```python
from build123d import *

# Parameters (mm, degrees)
CUT_EXTRUDE_1_DEPTH      = 5
EXTRUDE_1_DEPTH          = 6
PATTERN_CIRCULAR_1_COUNT = 3
SKETCH_4_R               = 42.404307435
SKETCH_4_R_2             = 25.5
CUT_EXTRUDE_2_DEPTH      = 9.5
CHAMFER_START            = 14
CHAMFER_1_DEPTH          = 6


with BuildPart() as part:
    # Эскиз1 → Повернуть1 (revolve)
    with BuildSketch(Plane.XY, mode=Mode.PRIVATE) as revolve_1_sk:
        with BuildLine():
            Line((-24, 0), (-24, 4.5))
            Line((-24, 4.5), (-25.5, 4.5))
            Line((-25.5, 4.5), (-25.5, 9.5))
            Line((-25.5, 9.5), (-19, 9.5))
            Line((-19, 9.5), (-19, 22))
            Line((-19, 22), (-24, 22))
            Line((-24, 22), (-24, 12.5))
            Line((-24, 12.5), (-27.5, 12.5))
            ThreePointArc((-27.5, 12.5), (-28.207106781, 12.207106781), (-28.5, 11.5))
            Line((-28.5, 11.5), (-28.5, 0))
            Line((-28.5, 0), (-24, 0))
        make_face()
    revolve(revolve_1_sk.sketch.rotate(Axis((0, 0, 0), (0, -1, 0)), 270), axis=Axis((0, 0, 0), (0, -1, 0)))

    # Эскиз2 → Вырез-Вытянуть1 (cut)
    with BuildSketch(Plane(origin=(0, 0, 0), x_dir=(-1, 0, 0), z_dir=(0, -1, 0))):
        with BuildLine():
            ThreePointArc((24, 0), (17.8818714, -16.007456864), (2.646777063, -23.85360709))
            Line((2.646777063, -23.85360709), (5, -25.514701644))
            ThreePointArc((5, -25.514701644), (20.0748599, -16.522711642), (26, 0))
            ThreePointArc((26, 0), (25.646694472, 4.271658071), (24.596379794, 8.427223803))
            Line((24.596379794, 8.427223803), (21.981218243, 9.63462737))
            ThreePointArc((21.981218243, 9.63462737), (23.489883331, 4.921928594), (24, 0))
        make_face()
        with BuildLine():
            Line((-5, -25.514701644), (-2.646777063, -23.85360709))
            ThreePointArc((-2.646777063, -23.85360709), (-20.784609691, -12), (-21.981218243, 9.63462737))
            Line((-21.981218243, 9.63462737), (-24.596379794, 8.427223803))
            ThreePointArc((-24.596379794, 8.427223803), (-22.516660498, -13), (-5, -25.514701644))
        make_face()
        with BuildLine():
            Line((-19.596379794, 17.087477841), (-19.33444118, 14.218979719))
            ThreePointArc((-19.33444118, 14.218979719), (0, 24), (19.33444118, 14.218979719))
            Line((19.33444118, 14.218979719), (19.596379794, 17.087477841))
            ThreePointArc((19.596379794, 17.087477841), (0, 26), (-19.596379794, 17.087477841))
        make_face()
    extrude(amount=-CUT_EXTRUDE_1_DEPTH, mode=Mode.SUBTRACT)

    # Эскиз3 → Бобышка-Вытянуть1 (add)
    with BuildSketch(Plane(origin=(25.5, 0, 0), x_dir=(0, 0, -1), z_dir=(1, 0, 0))):
        Polygon((-11.5, 20), (11.5, 20), (11.5, 17), (-11.5, 15), align=None)
    extrude_1 = extrude(amount=-EXTRUDE_1_DEPTH)

    # Круговой массив1: Бобышка-Вытянуть1 ×3 about axis
    pattern_circular_1_axis = Axis((0, 0, 0), (0, 1, 0))
    for i in range(1, PATTERN_CIRCULAR_1_COUNT):
        add(extrude_1.rotate(pattern_circular_1_axis, i * 360 / PATTERN_CIRCULAR_1_COUNT))

    # Эскиз4 → Вырез-Вытянуть2 (cut)
    with BuildSketch(Plane(origin=(0, 22, 0), x_dir=(1, 0, 0), z_dir=(0, 1, 0))):
        Circle(SKETCH_4_R)
        with Locations(Location((0, 0, 0), (0, 0, 270))):
            Circle(SKETCH_4_R_2, mode=Mode.SUBTRACT)
    extrude(amount=-CUT_EXTRUDE_2_DEPTH, mode=Mode.SUBTRACT)

    # Фаска1: read off the stored shape, not the designer's step
    # Фаска1 outline → Фаска1 (cut)
    with BuildSketch(Plane(origin=(0, 0, 0), x_dir=(1, 0, 0), z_dir=(0, 1, 0)).offset(CHAMFER_START)):
        with BuildLine():
            Line((-20.456443185, 12.551252218), (-20.356857991, 15.357354354))
            ThreePointArc((-20.356857991, 15.357354354), (-20.859675731, 14.667103612), (-21.33909882, 13.960403344))
            Line((-21.33909882, 13.960403344), (-20.49197936, 12.493149399))
            ThreePointArc((-20.49197936, 12.493149399), (-20.474231883, 12.522213414), (-20.456443185, 12.551252218))
        make_face()
        with BuildLine():
            ThreePointArc((-1.420514533, 25.460403344), (-2.272246462, 25.398560904), (-3.12143001, 25.308233338))
            Line((-3.12143001, 25.308233338), (-0.641481678, 23.991425578))
            ThreePointArc((-0.641481678, 23.991425578), (-0.607438987, 23.992311641), (-0.573395073, 23.993149399))
            Line((-0.573395073, 23.993149399), (-1.420514533, 25.460403344))
        make_face()
        with BuildLine():
            ThreePointArc((-20.456443185, -12.551252218), (-20.474231883, -12.522213414), (-20.49197936, -12.493149399))
            Line((-20.49197936, -12.493149399), (-21.33909882, -13.960403344))
            ThreePointArc((-21.33909882, -13.960403344), (-20.859675731, -14.667103612), (-20.356857991, -15.357354354))
            Line((-20.356857991, -15.357354354), (-20.456443185, -12.551252218))
        make_face()
        with BuildLine():
            Line((22.759613353, 11.5), (21.065374433, 11.5))
            ThreePointArc((21.065374433, 11.5), (21.08167087, 11.470098227), (21.097924862, 11.44017336))
            Line((21.097924862, 11.44017336), (23.478288, 9.950878984))
            ThreePointArc((23.478288, 9.950878984), (23.131922194, 10.731457292), (22.759613353, 11.5))
        make_face()
        with BuildLine():
            ThreePointArc((-0.573395073, -23.993149399), (-0.607438987, -23.992311641), (-0.641481678, -23.991425578))
            Line((-0.641481678, -23.991425578), (-3.12143001, -25.308233338))
            ThreePointArc((-3.12143001, -25.308233338), (-2.272246462, -25.398560904), (-1.420514533, -25.460403344))
            Line((-1.420514533, -25.460403344), (-0.573395073, -23.993149399))
        make_face()
        with BuildLine():
            ThreePointArc((22.759613353, -11.5), (23.131922194, -10.731457292), (23.478288, -9.950878984))
            Line((23.478288, -9.950878984), (21.097924862, -11.44017336))
            ThreePointArc((21.097924862, -11.44017336), (21.08167087, -11.470098227), (21.065374433, -11.5))
            Line((21.065374433, -11.5), (22.759613353, -11.5))
        make_face()
    extrude(amount=CHAMFER_1_DEPTH, mode=Mode.SUBTRACT)


solid = part.part
```
Read the model definition and answer for the solid it produces. Units are mm, in the model's axes. A direction names the side the tool comes from. Round coordinates to 2 decimals unless told otherwise and drop trailing zeros. One line per item, written item: value.
Q1. Which of the six approach directions +Z, -Z, +X, -X, +Y, -Y give full straight-line access (tool end or side, diameter ignored) to faces 5 (the flat face through (-12.3, 16, 21.3)), 6 (the cylindrical face through (-12.626, 18.142, -22.155)), 7 (the cylindrical face through (0, 2, 24)), 8 (the flat face through (0, 4.5, 25))?
Data:
face 5: +Z
face 6: -Z, -X, +Y
face 7: -Y
face 8: none
Q2. Straight lines are drawn through the part: line 1 (X direction, y = 15.5, z = 0); line 2 (X direction, y = 18.5, z = 0); line 3 (Y direction, x = 20.5, z = 14.5). For each, find the intervals that lie inside material, in ascending order. Write a range as [from, to].
Data:
line 1: [-24, -19], [19, 24]
line 2: [-24, -19], [19, 25.5]
line 3: [9.5, 12.5]
Q3. Flat-ended cylindrical pins translate along their axes: pin 1 Ø5 at (y, z) = (18, 21) entering from -X; pin 2 Ø2 at (x, z) = (-2.5, -16.5) entering from +Y; pin 3 Ø10 at (y, z) = (9.5, 15.5) entering from +X; pin 4 Ø0.5 at (x, z) = (-0.5, 24.5) entering from +Y. Find the tip coordinate at first contact, or state that the pin passes through.
Data:
pin 1: x = -17.55
pin 2: through
pin 3: x = 26.5
pin 4: y = 12.5
Q4. For a pull along X with two mould halves and no side action, classify faces 1 (the flat face through (23.27, 2.46, -9.04)), 2 (the cylindrical face through (22.67, 2.46, 12.73)), 3 (the cylindrical face through (-12.874, 18.142, 22.012)), 4 (the flat face through (-1.9, 17.47, -24.66)) as +X half, -X half, draft (parallel to the pull), parting line (faces both ways), or undercut.
Data:
face 1: undercut
face 2: undercut
face 3: -X half
face 4: +X half
